The model under review builds one solid part; all positions refer to its coordinate system, in mm. Round coordinates to 2 decimals unless told otherwise and drop trailing zeros. Write each loop counter-clockwise with the first axis right and the second up, starting at its lowest first coordinate (ties: lowest second). Pieces come first, ordered by that corner, then holes. Notation, with made-up numbers: (76, 14.25) -> (120, 14.25) arc R20 ccw to (120, 21.25) -> close; hole circle Ø1 at (32.25, 14). An arc over 180 degrees is marked (long way). Answer in a Markdown table with one row per item. Add a question column.
```python
from build123d import *

# Parameters (mm, degrees)
BOSS_EXTRUDE1_DEPTH = 3.175


with BuildPart() as part:
    # Sketch1 → Boss-Extrude1 (new body)
    with BuildSketch(Plane.XY):
        Polygon((38.1, 58.683525), (0, 58.683525), (0, 0), (450.85, 0), (450.85, 0.0254), (457.2, 0.0254), (457.2, 58.683525), (431.8, 58.683525), (431.8, 7.883525), (38.1, 7.883525), align=None)
        Polygon((0, 117.36705), (0, 58.683525), (38.1, 58.683525), (38.1, 109.483525), (431.8, 109.483525), (431.8, 58.683525), (457.2, 58.683525), (457.2, 117.34165), (450.85, 117.34165), (450.85, 117.36705), align=None)
    extrude(amount=BOSS_EXTRUDE1_DEPTH)


solid = part.part
```
1. Add section C-C on x = 269.5. Write out the cut boundary in (y, z) (3 decimals), plus the area to 3 significant figures.
2. For L1, parallel to Y at x = 231, z = 2.65; L2, parallel to X at y = 86, z = 2.2, list the stretches that pass through material, from the lowest coordinate up.
3. Add section A-A on y = 104. Write out the cut boundary in (x, z) (3 decimals).
Filled in:
| question | item | result |
|---|---|---|
| 1 | outline | (0, 0) -> (7.884, 0) -> (7.884, 3.175) -> (0, 3.175) -> close; (109.484, 0) -> (117.367, 0) -> (117.367, 3.175) -> (109.484, 3.175) -> close |
| 1 | area | 50.1 mm² |
| 2 | L1 | 0 to 7.88, 109.48 to 117.37 |
| 2 | L2 | 0 to 38.1, 431.8 to 457.2 |
| 3 | outline | (0, 0) -> (38.1, 0) -> (38.1, 3.175) -> (0, 3.175) -> close; (431.8, 0) -> (457.2, 0) -> (457.2, 3.175) -> (431.8, 3.175) -> close |
